The model under review builds one solid part; all positions refer to its coordinate system, in mm. Round coordinates to 2 decimals unless told otherwise and drop trailing zeros. Order: outer loops, then holes, each group sorted by start corner. A loop starts at its lowest first (then second) coordinate and runs counter-clockwise, first axis right, second up.
1) Consider section D-D (y = 68.25). Give the boundary of the cut face in (x, z).
2) Mouldability with a two-part tool opening along Y and no side actions: class faces 1 (the face through (-47.867, 67.095, 57.986)), 2 (the face through (-46, 73, 57)), 3 (the face through (-47, 73, 58)) as pulls with the +Y half, pulls with the -Y half, needs draft (parallel to the pull), parting line crosses it, or undercut.
3) Clearance check with a flat-ended pin moving along its axis: P1, Ø1, axis at x = -49.5, z = 58, coming from the -Y side. State where the tip first meets the part, or that it passes through.
4) To check wall thickness, follow L1, parallel to Y at x = -47, z = 58.6; L2, parallel to Y at x = -46.5, z = 57.15; L3, parallel to X at y = 69.25, z = 57.25. State the ranges of each line that lie inside material, in increasing order.
5) Consider section B-B (y = 71). Give the boundary of the cut face in (x, z).
6) Consider section C-C (z = 58). Give the boundary of the cut face in (x, y), then the cut area to 3 significant figures.
7) Consider section A-A (x = -47). Give the boundary of the cut face in (y, z).
from build123d import *

# Parameters (mm, degrees)
CYLINDER355_R     = 2
CYLINDER355_DEPTH = 2
CYLINDER356_R     = 4
CYLINDER356_DEPTH = 2


with BuildPart() as cylinder355:
    # Cylinder355 → Cylinder355 (new body)
    with BuildSketch(Plane.XY):
        Circle(CYLINDER355_R)
    extrude(amount=CYLINDER355_DEPTH)


with BuildPart() as spacer4:
    # Cylinder356 → Cylinder356 (new body)
    with BuildSketch(Plane.XY):
        Circle(CYLINDER356_R)
    extrude(amount=CYLINDER356_DEPTH)

    # Cut372: cut Cylinder355
    add(cylinder355.part, mode=Mode.SUBTRACT)


with BuildPart() as spacer4_1:
    # Cut372 placement: moved
    add(spacer4.part.moved(Location((-47, 71, 57))))


solid = spacer4_1.part
Answer below:
1. outline: (-49.9, 57) - (-44.1, 57) - (-44.1, 59) - (-49.9, 59) - close
2. face 1: parting line crosses it
2. face 2: needs draft
2. face 3: undercut
3. P1: stops at y = 67.54
4. L1: y = 67 to 69, 73 to 75
4. L2: y = 67.03 to 69.06, 72.94 to 74.97
4. L3: x = -50.6 to -47.97, -46.03 to -43.4
5. outline: (-51, 57) - (-49, 57) - (-49, 59) - (-51, 59) - close; (-45, 57) - (-43, 57) - (-43, 59) - (-45, 59) - close
6. outline: circle Ø8 at (-47, 71); hole circle Ø4 at (-47, 71)
6. area: 37.7 mm2
7. outline: (67, 57) - (69, 57) - (69, 59) - (67, 59) - close; (73, 57) - (75, 57) - (75, 59) - (73, 59) - close
